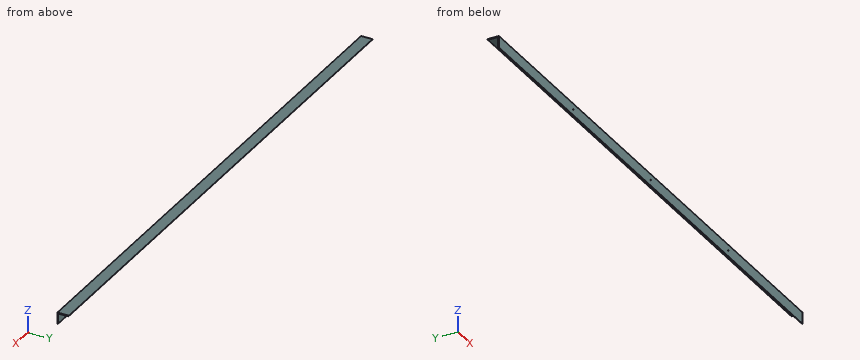
```python
from build123d import *

# Parameters (mm, degrees)
L_ANGLE_EQUAL_40X40X3_2_DEPTH = 1920
SKETCH15_R                    = 2
CUT_EXTRUDE1_DEPTH            = 10


with BuildPart() as part:
    # Sketch13 → L angle (equal) 40X40X3(2) (new body)
    with BuildSketch(Plane(origin=(0, 0, 0), x_dir=(0, 0, -1), z_dir=(1, 0, 0))):
        with BuildLine():
            Line((0, 40), (0, 0))
            Line((0, 0), (40, 0))
            ThreePointArc((40, 0), (39.121320344, 2.121320344), (37, 3))
            Line((37, 3), (9, 3))
            ThreePointArc((9, 3), (4.757359313, 4.757359313), (3, 9))
            Line((3, 9), (3, 37))
            ThreePointArc((3, 37), (2.121320344, 39.121320344), (0, 40))
        make_face()
    extrude(amount=L_ANGLE_EQUAL_40X40X3_2_DEPTH)

    # Sketch15 → Cut-Extrude1 (cut)
    with BuildSketch(Plane(origin=(0, 0, 0), x_dir=(-1, 0, 0), z_dir=(0, -1, 0))):
        with Locations(Location((-960, 20, 0), (0, 0, 90))):
            Circle(SKETCH15_R)
        with Locations(Location((-470, 20, 0), (0, 0, 90))):
            Circle(SKETCH15_R)
        with Locations(Location((-1450, 20, 0), (0, 0, 90))):
            Circle(SKETCH15_R)
    extrude(amount=-CUT_EXTRUDE1_DEPTH, mode=Mode.SUBTRACT)


solid = part.part
```
Verification items for the finished model (mm, model axes). Give positions to 0.01 mm unless a question says otherwise; leave off trailing zeros. Order: outer loops, then holes, each group sorted by start corner. A loop starts at its lowest first (then second) coordinate and runs counter-clockwise, first axis right, second up. Notation, with made-up numbers: M -16,27 L 12,27 A26 ccw 12,46 Z; hole C -21,-1.75 d6. An arc over 180 degrees is marked long. Return JSON: item names as keys, results as strings. Group by question number.
1) Section check A-A on x = 366. Record the cut outline in (y, z), and give its area (3 significant figures).
2) Scan lines: line 1 (X direction, y = 1, z = -20); line 2 (Z direction, x = 470, y = 0.85); line 3 (Z direction, x = 470, y = 1.2). Record each from-to range of solid material in increasing order.
3) Section check B-B on y = 19. Record the cut outline in (x, z).
4) Go/stop test with flat-tipped pins: pin 1 Ø3 at (x, y) = (312.5, 5) entering from -Z; pin 2 Ø14 at (x, z) = (1312, -20.5) entering from +Y; pin 3 Ø4 at (x, y) = (1168, 27) entering from -Z. Record where each tip stops, or that it passes through.
Answer block:
{
 "1": {"outline": "M 0,-40 A3 ccw 3,-37 L 3,-9 A6 cw 9,-3 L 37,-3 A3 ccw 40,0 L 0,0 Z", "area": "235 mm^2"},
 "2": {"line 1": "x = 0 to 468, 472 to 958, 962 to 1448, 1452 to 1920", "line 2": "z = -39.88 to -22, -18 to 0", "line 3": "z = -39.75 to -22, -18 to 0"},
 "3": {"outline": "M 0,-3 L 1920,-3 L 1920,0 L 0,0 Z"},
 "4": {"pin 1": "stops at z = -6.6", "pin 2": "stops at y = 3", "pin 3": "stops at z = -3"}
}
